Build history of the part. All positions in model axes, mm. Round coordinates to 2 decimals unless told otherwise and drop trailing zeros. Write each loop counter-clockwise with the first axis right and the second up, starting at its lowest first coordinate (ties: lowest second). Pieces come first, ordered by that corner, then holes. Notation, with made-up numbers: (-29, 47.25) - (-17, 47.25) arc R35 ccw to (-17, 79.25) - close; hole circle Ø7 at (73, -4). An arc over 180 degrees is marked (long way). Answer as a JSON object with one key per item and string values. Group by question number.
Item 1: Flat gauge pin, fed straight in: pin 1 (3 mm diameter, centred on x = 0, y = 13.725, fed in from -Z). Where does the tip first touch, or does it go through?
Item 2: Probe line 1 (Y direction, x = 0, z = 2.7) (3 decimals); line 2 (Y direction, x = -1.25, z = 2.45) (3 decimals); line 3 (X direction, y = 13, z = 4.5). List the from-to ranges inside material, lowest first. Write a range as from..to.
Item 3: Slice it at A-A, the plane y = 13. List the corners of the cut face in (x, z), then the cut area to 3 significant figures.
Item 4: Slice it at C-C, the plane z = 2.6. Give the number of separate pieces and of enclosed holes in the cut face, then the cut area to 3 significant figures.
Item 5: Two-plate mould, pull along Y, no slides. Class faces 1 (the cylindrical face through (3.496, 17.299, 2.535)), 2 (the flat face through (0, 0, 5)), 3 (the cylindrical face through (-0.33, 2.31, 2.46)), 4 (the cylindrical face through (-0.33, -5.19, 2.46)): +Y half, -Y half, draft (parallel to the pull), parting line (faces both ways), or undercut.
Item 6: Slice it at B-B, the plane x = 1. List the corners of the cut face in (y, z) (3 decimals), then the cut area to 3 significant figures.
from build123d import *

# Parameters (mm, degrees)
SKETCH_1_W      = 10
SKETCH_1_H      = 37.45
SKETCH_1_R      = 1.5
SKETCH_1_R_2    = 2
EXTRUDE_1_DEPTH = 5
FILLET_1_R      = 5
FILLET_2_R      = 3


with BuildPart() as part:
    # ｽｹｯﾁ1 → ﾎﾞｽ - 押し出し1 (new body)
    with BuildSketch(Plane.XY):
        Rectangle(SKETCH_1_W, SKETCH_1_H)
        with Locations((0, -13.725)):
            Circle(SKETCH_1_R, mode=Mode.SUBTRACT)
        with Locations((0, -3.725)):
            Circle(SKETCH_1_R, mode=Mode.SUBTRACT)
        with Locations((0, 13.725)):
            Circle(SKETCH_1_R_2, mode=Mode.SUBTRACT)
        with Locations((0, 3.775)):
            Circle(SKETCH_1_R, mode=Mode.SUBTRACT)
    extrude(amount=EXTRUDE_1_DEPTH)

    # ﾌｨﾚｯﾄ1
    fillet_1_edges = [part.edges().sort_by_distance(p)[0] for p in [
        (5, 18.725, 2.5),
        (-5, 18.725, 2.5),
    ]]
    fillet(fillet_1_edges, radius=FILLET_1_R - 0.0001)  # a hair under: the kernel refuses the full size

    # ﾌｨﾚｯﾄ2
    fillet_2_edges = [part.edges().sort_by_distance(p)[0] for p in [
        (5, -18.725, 2.5),
        (-5, -18.725, 2.5),
    ]]
    fillet(fillet_2_edges, radius=FILLET_2_R)


solid = part.part
Geometry says:
{
 "1": {"pin 1": "passes through"},
 "2": {"line 1": "y = -18.725..-15.225, -12.225..-5.225, -2.225..2.275, 5.275..11.725, 15.725..18.725", "line 2": "y = -18.725..-14.554, -12.896..-4.554, -2.896..2.946, 4.604..12.164, 15.286..18.566", "line 3": "x = -5..-1.86, 1.86..5"},
 "3": {"outline": "(-5, 0) - (-1.86, 0) - (-1.86, 5) - (-5, 5) - close; (1.86, 0) - (5, 0) - (5, 5) - (1.86, 5) - close", "area": "31.4 mm^2"},
 "4": {"separate pieces": "1", "enclosed holes": "4", "area": "326 mm^2"},
 "5": {"face 1": "+Y half", "face 2": "draft", "face 3": "undercut", "face 4": "undercut"},
 "6": {"outline": "(-18.725, 0) - (-14.843, 0) - (-14.843, 5) - (-18.725, 5) - close; (-12.607, 0) - (-4.843, 0) - (-4.843, 5) - (-12.607, 5) - close; (-2.607, 0) - (2.657, 0) - (2.657, 5) - (-2.607, 5) - close; (4.893, 0) - (11.993, 0) - (11.993, 5) - (4.893, 5) - close; (15.457, 0) - (18.624, 0) - (18.624, 5) - (15.457, 5) - close", "area": "136 mm^2"}
}
